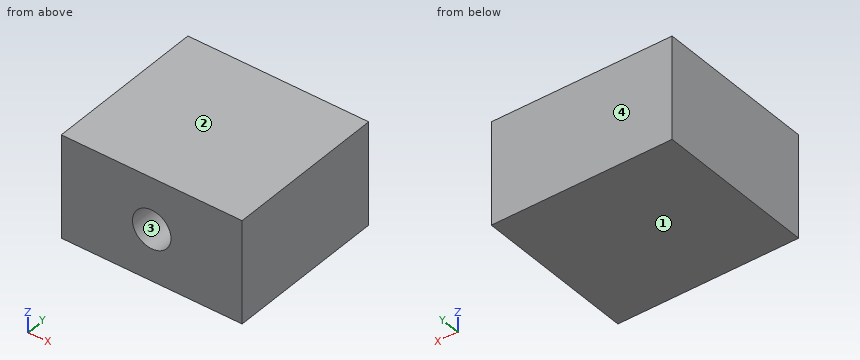
from build123d import *

# Parameters (mm, degrees)
SKETCH1_W      = 22.352
SKETCH1_H      = 20.066
EXTRUDE1_DEPTH = 6.35
SKETCH2_R      = 2.38125
EXTRUDE2_DEPTH = 12.7


with BuildPart() as part:
    # Sketch1 → Extrude1 (new body, symmetric)
    with BuildSketch(Plane.XY):
        Rectangle(SKETCH1_W, SKETCH1_H)
    extrude(amount=EXTRUDE1_DEPTH, both=True)

    # Sketch2 → Extrude2 (cut)
    with BuildSketch(Plane.XZ.offset(10.033)):
        with Locations(Location((0, 0, 0), (0, 0, 270))):  # turned: the seam where the file's is
            Circle(SKETCH2_R)
    extrude(amount=-EXTRUDE2_DEPTH, mode=Mode.SUBTRACT)


solid = part.part
Geometry: final body of the model. Coordinates: model frame, mm. Face numbers are marked on the shaded views. Coordinates: 2 decimals unless noted, no trailing zeros. Order: outer loops, then holes, each group sorted by start corner. A loop starts at its lowest first (then second) coordinate and runs counter-clockwise, first axis right, second up. Notation, with made-up numbers: (14, 66) - (37, 66) arc R18 ccw to (37, 88) - close; hole circle Ø6 at (61, 70). An arc over 180 degrees is marked (long way). Use one line per item in the form item = value.
1) Section C-C (z = 0). Return loops of the section in (x, y).
Solutions:
outline = (-11.18, -10.03) - (-2.38, -10.03) - (-2.38, 2.67) - (2.38, 2.67) - (2.38, -10.03) - (11.18, -10.03) - (11.18, 10.03) - (-11.18, 10.03) - close
2) Mould query, pull axis Z, two halves, no side actions, for the marked faces 1, 2, 3 and 4. Classes: +Z half, -Z half, draft (parallel to the pull), parting line (faces both ways), or undercut.
Solutions:
face_1 = -Z half
face_2 = +Z half
face_3 = undercut
face_4 = draft
3) Ray query, L1, parallel to X at y = -0.25, z = 0; L2, parallel to X at y = -9, z = -1.25; L3, parallel to Z at x = 1.5, y = -1.5. Return the intervals inside material, ascending.
Solutions:
L1 = -11.18 to -2.38, 2.38 to 11.18
L2 = -11.18 to -2.03, 2.03 to 11.18
L3 = -6.35 to -1.85, 1.85 to 6.35
4) Section A-A (y = 0.25). Return loops of the section in (x, z).
Solutions:
outline = (-11.18, -6.35) - (11.18, -6.35) - (11.18, 6.35) - (-11.18, 6.35) - close; hole circle Ø4.76 at (0, 0)
5) Pin query (flat end, axial travel): pin 1 (4 mm diameter, centred on x = 0.5, z = -1, fed in from -Y). Return the tip coordinate at first contact, or that it passes through.
Solutions:
pin_1 = -10.03
6) Section B-B (x = 0). Return loops of the section in (y, z), then the cut area to 3 significant figures.
Solutions:
outline = (-10.03, -6.35) - (10.03, -6.35) - (10.03, 6.35) - (-10.03, 6.35) - (-10.03, 2.38) - (2.67, 2.38) - (2.67, -2.38) - (-10.03, -2.38) - close
area = 194 mm^2
